Read the model definition and answer for the solid it produces. Units are mm, in the model's axes. Face numbers are marked on the shaded views. A direction names the side the tool comes from. Coordinates: 2 decimals unless noted, no trailing zeros. Write each loop counter-clockwise with the first axis right and the second up, starting at its lowest first coordinate (ties: lowest second). Pieces come first, ordered by that corner, then holes.
Item 1: Section B-B (x = 15) is taken. Give the vertices of the cut face in (y, z).
Item 2: Straight lines are drawn through the part: probe 1 along Z at (x, y) = (15.75, -6.75); probe 2 along X at (y, z) = (-3.5, 5.75); probe 3 along X at (y, z) = (-16.5, 8). For each, find the intervals that lie inside material, in ascending order.
Item 3: A tool of negligible diameter and unlimited length cuts with its end or side. For the marked faces 1, 2, 3, 4 and 5, from which of +Z, -Z, +X, -X, +Y, -Y can it reach the whole face along a straight path? Write none if from no direction.
Item 4: Each of these flat-tipped pins is pushed along its axis until it touches: P1, Ø1, axis at y = -5.5, z = 5.5, coming from the -X side; P2, Ø2, axis at y = -17.5, z = 9.5, coming from the +X side; P3, Ø2, axis at x = 12, z = 6, coming from the +Y side; P4, Ø0.9, axis at x = 16, y = -14, coming from the +Z side. Where does it stop, or does it pass through?
Item 5: Section A-A (y = -9) is taken. Give the vertices of the cut face in (x, z).
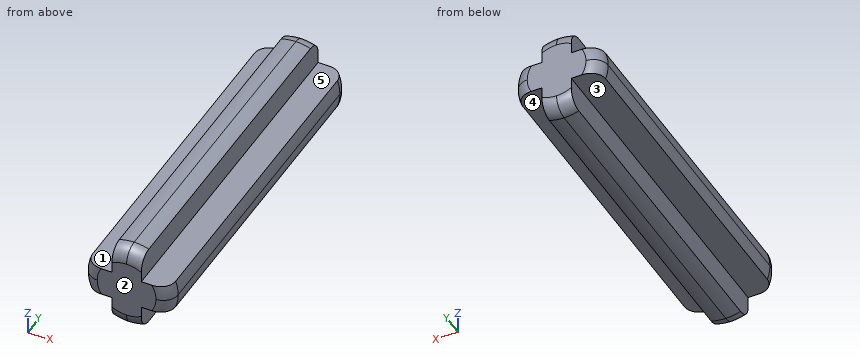
from build123d import *

# Parameters (mm, degrees)
F0_W     = 2
F0_H     = 2
F1_DEPTH = 23.4
F2_R     = 1


with BuildPart() as f1:
    # F0 (on Front) → F1 (new body)
    with BuildSketch(Plane.XZ):
        with BuildLine():
            Line((12.5810803622, 6.8602320091), (12.5810803622, 8.8602320091))
            Line((12.5810803622, 8.8602320091), (10.7526532375, 8.8602320091))
            ThreePointArc((10.7526532375, 8.8602320091), (10.6242846832, 8.3675379453), (10.5810803622, 7.8602320091))
            ThreePointArc((10.5810803622, 7.8602320091), (10.6242846832, 7.3529260729), (10.7526532375, 6.8602320091))
            Line((10.7526532375, 6.8602320091), (12.5810803622, 6.8602320091))
        make_face()
        with Locations((13.5810803622, 7.8602320091)):
            Rectangle(F0_W, F0_H)
        with BuildLine():
            Line((14.5810803622, 8.8602320091), (14.5810803622, 10.6886591338))
            ThreePointArc((14.5810803622, 10.6886591338), (14.0883862984, 10.8170276881), (13.5810803622, 10.8602320091))
            ThreePointArc((13.5810803622, 10.8602320091), (13.073774426, 10.8170276881), (12.5810803622, 10.6886591338))
            Line((12.5810803622, 10.6886591338), (12.5810803622, 8.8602320091))
            Line((12.5810803622, 8.8602320091), (14.5810803622, 8.8602320091))
        make_face()
        with BuildLine():
            ThreePointArc((13.5810803622, 4.8602320091), (14.0883862984, 4.9034363301), (14.5810803622, 5.0318048844))
            Line((14.5810803622, 5.0318048844), (14.5810803622, 6.8602320091))
            Line((14.5810803622, 6.8602320091), (12.5810803622, 6.8602320091))
            Line((12.5810803622, 6.8602320091), (12.5810803622, 5.0318048844))
            ThreePointArc((12.5810803622, 5.0318048844), (13.073774426, 4.9034363301), (13.5810803622, 4.8602320091))
        make_face()
        with BuildLine():
            ThreePointArc((16.4095074869, 6.8602320091), (16.5378760412, 7.3529260729), (16.5810803622, 7.8602320091))
            ThreePointArc((16.5810803622, 7.8602320091), (16.5378760412, 8.3675379453), (16.4095074869, 8.8602320091))
            Line((16.4095074869, 8.8602320091), (14.5810803622, 8.8602320091))
            Line((14.5810803622, 8.8602320091), (14.5810803622, 6.8602320091))
            Line((14.5810803622, 6.8602320091), (16.4095074869, 6.8602320091))
        make_face()
    extrude(amount=F1_DEPTH)

    # F2
    f2_edges = [f1.edges().sort_by_distance(p)[0] for p in [
        (16.58108, 0, 7.860232),
        (13.58108, 0, 10.860232),
        (10.58108, 0, 7.860232),
        (13.58108, 0, 4.860232),
        (13.58108, -23.4, 10.860232),
        (10.58108, -23.4, 7.860232),
        (13.58108, -23.4, 4.860232),
        (16.58108, -23.4, 7.860232),
    ]]
    fillet(f2_edges, radius=F2_R)


solid = f1.part
Established:
1. outline: (-23.4, 6.86) - (0, 6.86) - (0, 8.86) - (-23.4, 8.86) - close
2. probe 1: z = 6.86 to 8.86
2. probe 2: x = 12.58 to 14.58
2. probe 3: x = 10.58 to 16.58
3. face 1: +Z, -X, +Y, -Y
3. face 2: +Z, -Z, +X, -X, -Y
3. face 3: -Z, -X, +Y, -Y
3. face 4: -Z, +X, +Y, -Y
3. face 5: +Z, +X, +Y, -Y
4. P1: stops at x = 12.58
4. P2: stops at x = 16.51
4. P3: stops at y = 0
4. P4: stops at z = 8.86
5. outline: (10.75, 6.86) - (12.58, 6.86) - (12.58, 5.03) arc R3 ccw to (14.58, 5.03) - (14.58, 6.86) - (16.41, 6.86) arc R3 ccw to (16.41, 8.86) - (14.58, 8.86) - (14.58, 10.69) arc R3 ccw to (12.58, 10.69) - (12.58, 8.86) - (10.75, 8.86) arc R3 ccw to start
